The model under review builds one solid part; all positions refer to its coordinate system, in mm. A direction names the side the tool comes from. Round coordinates to 2 decimals unless told otherwise and drop trailing zeros. Write each loop counter-clockwise with the first axis right and the second up, starting at its lowest first coordinate (ties: lowest second). Pieces come first, ordered by that corner, then holes. Notation, with made-up numbers: (-28.5, 21) - (-19.5, 21) arc R10 ccw to (-19.5, 34) - close; hole circle Ø11 at (76.25, 63). An arc over 180 degrees is marked (long way). Return JSON: item names as keys, results as strings.
from build123d import *

# Parameters (mm, degrees)
F0_W        = 580
F0_H        = 540
F1_DEPTH    = 7.5
F2_T        = -20
F3_T1_DEPTH = 695.9123277853
F3_T3_DEPTH = 735.9123277853
F4_R        = 2
F5_W        = 540
F5_H        = 500
F6_DEPTH    = 4


# Not quite as in the source:
# - a fillet or chamfer that OpenCascade refuses, or shapes differently, is made with other operations: its cross-section is extruded or revolved along the edge and cut away or added


with BuildPart() as f1:
    # F0 (on Top) → F1 (new body)
    with BuildSketch(Plane.XY):
        with Locations((-1.4553386718, -5.8427717585)):
            Rectangle(F0_W, F0_H)
    extrude(amount=F1_DEPTH)

    # F2
    f2_openings = [f1.faces().sort_by_distance(p)[0] for p in [
        (-1.455339, -5.842772, 7.5),
        (-1.455339, -5.842772, 0),
    ]]
    offset(amount=F2_T, openings=f2_openings)

    # F3: chamfer of 30 x 5.2898094213 on 4 edges, made by hand

    # F3_s2 → F3_t1 (cut)
    with BuildSketch(Plane.XZ.offset(-342.1133921341)):
        Polygon((-291.4553386718, 2.2101905787), (-261.4553386718, 7.5), (-291.4553386718, 7.5), align=None)
        Polygon((288.5446613282, 2.2101905787), (258.5446613282, 7.5), (288.5446613282, 7.5), align=None)
    extrude(amount=F3_T1_DEPTH, mode=Mode.SUBTRACT)

    # F3_s4 → F3_t3 (cut)
    with BuildSketch(Plane.YZ.offset(-369.4115025644)):
        Polygon((-275.8427717585, 2.2101905787), (-245.8427717585, 7.5), (-275.8427717585, 7.5), align=None)
        Polygon((264.1572282415, 2.2101905787), (234.1572282415, 7.5), (264.1572282415, 7.5), align=None)
    extrude(amount=F3_T3_DEPTH, mode=Mode.SUBTRACT)

    # F4
    f4_edges = [f1.edges().sort_by_distance(p)[0] for p in [
        (-291.455339, -5.842772, 2.210191),
        (-1.455339, -275.842772, 2.210191),
        (288.544661, -5.842772, 2.210191),
        (-1.455339, 264.157228, 2.210191),
    ]]
    fillet(f4_edges, radius=F4_R)

    # F5 (on Top) → F6 (join)
    with BuildSketch(Plane.XY):
        with Locations((-1.4553386718, -5.8427717585)):
            Rectangle(F5_W, F5_H)
    extrude(amount=F6_DEPTH)


solid = f1.part
(1) Add section A-A (x = 97). Write out the cut boundary in (y, z).
Filled in:
{"outline": "(-275.84, 0) - (264.16, 0) - (264.16, 0.53) arc R2 ccw to (262.5, 2.5) - (244.16, 5.74) - (244.16, 4) - (-255.84, 4) - (-255.84, 5.74) - (-274.19, 2.5) arc R2 ccw to (-275.84, 0.53) - close"}
(2) For faces 1 (the flat face through (-5.492, 253.459, 4.097)), 2 (the flat face through (-5, -2, 4)), list the 3-axis set-ups (+Z, -Z, +X, -X, +Y, -Y) from which the entire face can be reached by the end or side of a thin tool; tool diameter is ignored.
Filled in:
{"face 1": "+Z, +X, -X, +Y", "face 2": "+Z"}
(3) Wall thickness on line 1 (Z direction, x = 168.5, y = 15); line 2 (Y direction, x = -42, z = 1.1); line 3 (X direction, y = 44, z = 2.35): over which ranges is each line inside the solid? List them lowest first.
Filled in:
{"line 1": "z = 0 to 4", "line 2": "y = -275.76 to 264.07", "line 3": "x = -290.29 to 287.38"}
(4) Clearance check with flat-ended pins moving along their axes: pin 1 Ø2 at (x, z) = (-129, 2.5) entering from -Y; pin 2 Ø4 at (x, y) = (-144, 134) entering from +Z. State where each tip first meets the part, or that it passes through.
Filled in:
{"pin 1": "stops at y = -275.59", "pin 2": "stops at z = 4"}
(5) Add section B-B (y = -150). Write out the cut boundary in (x, z), plus the area to 3 significant figures.
Filled in:
{"outline": "(-291.46, 0) - (288.54, 0) - (288.54, 0.53) arc R2 ccw to (286.89, 2.5) - (268.54, 5.74) - (268.54, 4) - (-271.46, 4) - (-271.46, 5.74) - (-289.8, 2.5) arc R2 ccw to (-291.46, 0.53) - close", "area": "2,320 mm2"}
